```python
from build123d import *

# Parameters (mm, degrees)
F0_R         = 25.4
F1_DEPTH     = 6.35
F2_R         = 23.8125
F3_DEPTH     = 12.7
F4_R         = 25.4
F5_DEPTH     = 6.35
F6_S7_R      = 23.8125
F6_T8_DEPTH  = 40
F6_S13_R     = 23.8125
F6_T14_DEPTH = 40
F7_R         = 2.2698789725
F8_DEPTH     = 3.175
F9_R         = 6.35
F10_DEPTH    = 25.401


# Not quite as in the source:
# - a fillet or chamfer that OpenCascade refuses, or shapes differently, is made with other operations: its cross-section is extruded or revolved along the edge and cut away or added


with BuildPart() as f1:
    # F0 (on Front) → F1 (new body)
    with BuildSketch(Plane.XZ):
        Circle(F0_R)
    extrude(amount=F1_DEPTH)

    # F2 (on face) → F3 (join)
    with BuildSketch(Plane.XZ.offset(6.35)):
        Circle(F2_R)
    extrude(amount=F3_DEPTH)

    # F4 (on face) → F5 (join)
    with BuildSketch(Plane.XZ.offset(19.05)):
        Circle(F4_R)
    extrude(amount=F5_DEPTH)

    # F6: fillet of radius 1.6002 on 4 edges, made by hand

    # F6_s1 → F6_t2 (revolve, cut)
    with BuildSketch(Plane.XY):
        with BuildLine():
            ThreePointArc((25.4, -23.7998), (24.9313122713, -24.9313122713), (23.7998, -25.4))
            Line((23.7998, -25.4), (25.4, -25.4))
            Line((25.4, -25.4), (25.4, -23.7998))
        make_face()
    revolve(axis=Axis((0, -25.4, 0), (0, -1, 0)), mode=Mode.SUBTRACT)


with BuildPart() as f6_tool4:
    # F6_s5 → F6_t6 (revolve)
    with BuildSketch(Plane.XY):
        with BuildLine():
            ThreePointArc((25.4, -20.6502), (24.9313122713, -19.5186877287), (23.7998, -19.05))
            Line((23.7998, -19.05), (25.4, -19.05))
            Line((25.4, -19.05), (25.4, -20.6502))
        make_face()
    revolve(axis=Axis((0, -19.05, 0), (0, -1, 0)))

    # F6_s7 → F6_t8 (cut, symmetric)
    with BuildSketch(Plane.XZ.offset(19.9)):
        Circle(F6_S7_R)
    extrude(amount=F6_T8_DEPTH, both=True, mode=Mode.SUBTRACT)


with BuildPart() as f1_1:
    add(f1.part)

    # F6_t3: cut F6_tool4
    add(f6_tool4.part, mode=Mode.SUBTRACT)


with BuildPart() as f6_tool10:
    # F6_s11 → F6_t12 (revolve)
    with BuildSketch(Plane.XY):
        with BuildLine():
            ThreePointArc((23.7998, -6.35), (24.9313122713, -5.8813122713), (25.4, -4.7498))
            Line((25.4, -4.7498), (25.4, -6.35))
            Line((25.4, -6.35), (23.7998, -6.35))
        make_face()
    revolve(axis=Axis((0, -6.35, 0), (0, -1, 0)))

    # F6_s13 → F6_t14 (cut, symmetric)
    with BuildSketch(Plane.XZ.offset(5)):
        Circle(F6_S13_R)
    extrude(amount=F6_T14_DEPTH, both=True, mode=Mode.SUBTRACT)


with BuildPart() as f1_2:
    add(f1_1.part)

    # F6_t9: cut F6_tool10
    add(f6_tool10.part, mode=Mode.SUBTRACT)

    # F6_s15 → F6_t16 (revolve, cut)
    with BuildSketch(Plane.XY):
        with BuildLine():
            ThreePointArc((25.4, -1.6002), (24.9313122713, -0.4686877287), (23.7998, 0))
            Line((23.7998, 0), (25.4, 0))
            Line((25.4, 0), (25.4, -1.6002))
        make_face()
    revolve(axis=Axis((0, 0, 0), (0, -1, 0)), mode=Mode.SUBTRACT)

    # F7 (on face) → F8 (cut)
    with BuildSketch(Plane.XZ.offset(25.4)):
        with Locations((-19.05, 0)):
            Circle(F7_R)
        with Locations((0, -19.05)):
            Circle(F7_R)
        with Locations((19.05, 0)):
            Circle(F7_R)
        with Locations((0, 19.05)):
            Circle(F7_R)
    extrude(amount=-F8_DEPTH, mode=Mode.SUBTRACT)

    # F9 (on face) → F10 (cut, through all)
    with BuildSketch(Plane.XZ.offset(25.4)):
        Circle(F9_R)
    extrude(amount=-F10_DEPTH, mode=Mode.SUBTRACT)


solid = f1_2.part
```
Model file for the job. Use its own axes, mm. A direction names the side the tool comes from. Give positions to 0.01 mm unless a question says otherwise; leave off trailing zeros. Order: outer loops, then holes, each group sorted by start corner. A loop starts at its lowest first (then second) coordinate and runs counter-clockwise, first axis right, second up.
1) 3-axis set-ups, long thin cutter, end or side, ignore diameter. For faces 5 (the cylindrical face through (-5.506, -22.203, -24.796)), 6 (the flat face through (19, -22.225, 0)): which of +Z, -Z, +X, -X, +Y, -Y reach the whole face in a straight line?
2) Mould opens along Z. For faces 1 (the flat face through (5, -25.4, -5)), 2 (the flat face through (-19, -22.225, 0)), 3 (the cylindrical face through (-0.492, -23.835, -21.266)), 4 (the cylindrical face through (-5.506, -3.153, -24.796)) say: +Z half, -Z half, draft (parallel to the pull), parting line (faces both ways), or undercut.
3) Pin check, flat tips, straight feed: pin 1 (5 mm diameter, centred on y = -9, z = 8, fed in from -X); pin 2 (1.5 mm diameter, centred on y = -22, z = -14, fed in from -X); pin 3 (10 mm diameter, centred on x = 12, y = -11.5, fed in from +Z). Stop position of each tip, or through.
4) Wall check: probe 1 along Z at (x, y) = (0, -16); probe 2 along X at (y, z) = (-17.75, 3); probe 3 along Z at (x, y) = (5.5, -17.5). Give the ranges that are in metal, low to high.
5) Saw through at C-C, the plane y = -2.5. Write the cut outline in (x, z), then the cut area to 3 significant figures.
Computed:
1. face 5: +Y, -Y
1. face 6: -Y
2. face 1: draft
2. face 2: undercut
2. face 3: undercut
2. face 4: parting line
3. pin 1: stops at x = -23.17
3. pin 2: stops at x = -21.67
3. pin 3: stops at z = 22.76
4. probe 1: z = -23.81 to -6.35, 6.35 to 23.81
4. probe 2: x = -23.62 to -5.6, 5.6 to 23.62
4. probe 3: z = -23.17 to -3.17, 3.17 to 23.17
5. outline: circle Ø50.8 at (0, 0); hole circle Ø12.7 at (0, 0)
5. area: 1,900 mm2
